Input: part model. Units: mm. Frame: model coordinates. Give positions to 0.01 mm unless a question says otherwise; leave off trailing zeros. Order: outer loops, then holes, each group sorted by start corner. A loop starts at its lowest first (then second) coordinate and runs counter-clockwise, first axis right, second up. Notation, with made-up numbers: (-8.5, 58.5) - (46.5, 58.5) arc R20 cw to (46.5, 81.5) - close; hole circle Ø9 at (8, 10). An arc over 180 degrees is marked (long way). Use a Markdown table: item, result.
from build123d import *

# Parameters (mm, degrees)
BOSS_EXTRUDE1_DEPTH      = 60
SKETCH3_W                = 20
SKETCH3_H                = 20
SKETCH3_W_2              = 18
SKETCH3_H_2              = 18
BOSS_EXTRUDE2_DEPTH      = 2000
BOSS_EXTRUDE2_DEPTH_BACK = 20
CUT_EXTRUDE1_DEPTH       = 60
SKETCH7_W                = 200
SKETCH7_H                = 200
BOSS_EXTRUDE3_DEPTH      = 4
SKETCH8_W                = 109.20231627
SKETCH8_H                = 482.966945154
CUT_EXTRUDE3_DEPTH       = 1000
CUT_EXTRUDE4_REACH       = 29
SKETCH9_R                = 3.999999996
CUT_EXTRUDE5_REACH       = 52
SKETCH10_R               = 4.000000003
CUT_EXTRUDE6_REACH       = 1055.099
SKETCH11_R               = 5
FILLET1_R                = 2
FILLET2_R                = 2


with BuildPart() as part:
    # Sketch1 → Boss-Extrude1 (new body)
    with BuildSketch(Plane(origin=(0, 0, 0), x_dir=(0, 0, -1), z_dir=(1, 0, 0))):
        Polygon((0, 0), (0, 50), (-4, 50), (-4, 4), (-27, 4), (-27, 0), align=None)
    extrude(amount=BOSS_EXTRUDE1_DEPTH)

    # Sketch3 → Boss-Extrude2 (add, two sides)
    with BuildSketch(Plane(origin=(0.734152256, 4.01424851, 2.317627458), x_dir=(0, -0.5, 0.866025404), z_dir=(-0.156434465, -0.855363194, -0.49384417))) as boss_extrude2_sk:
        with Locations((0, -29.630650218)):
            Rectangle(SKETCH3_W, SKETCH3_H)
        with Locations((0, -29.630650218)):
            Rectangle(SKETCH3_W_2, SKETCH3_H_2, mode=Mode.SUBTRACT)
    extrude(amount=BOSS_EXTRUDE2_DEPTH)
    extrude(boss_extrude2_sk.sketch, amount=-BOSS_EXTRUDE2_DEPTH_BACK)

    # Sketch5 → Cut-Extrude1 (cut)
    with BuildSketch(Plane.ZY):
        Polygon((4, 4), (4, 36.054903459), (38.781358344, 4), align=None)
    extrude(amount=-CUT_EXTRUDE1_DEPTH, mode=Mode.SUBTRACT)

    # Sketch7 → Boss-Extrude3 (add)
    with BuildSketch(Plane(origin=(-155.547262091, -982.086761679, 2e-09), x_dir=(0.987688341, -0.156434465, 0), z_dir=(0.156434465, 0.987688341, 0))):
        with Locations((5.477031178, 566.441418592)):
            Rectangle(SKETCH7_W, SKETCH7_H)
    extrude(amount=BOSS_EXTRUDE3_DEPTH)

    # Sketch8 → Cut-Extrude3 (cut)
    with BuildSketch(Plane(origin=(-155.547262091, -982.086761679, 2e-09), x_dir=(0.987688341, -0.156434465, 0), z_dir=(-0.156434465, -0.987688341, 0))):
        with Locations((4.33544583, -787.065663544)):
            Rectangle(SKETCH8_W, SKETCH8_H)
    extrude(amount=CUT_EXTRUDE3_DEPTH, mode=Mode.SUBTRACT)

    # Sketch9 → Cut-Extrude4 (cut, up to next)
    with BuildSketch(Plane(origin=(0, 0, 0), x_dir=(-1, 0, 0), z_dir=(0, 0, -1)), mode=Mode.PRIVATE) as cut_extrude4_sk1:
        with Locations((-50, 22)):
            Circle(SKETCH9_R)
    cut_extrude4_tool1 = extrude(cut_extrude4_sk1.sketch, amount=-CUT_EXTRUDE4_REACH, mode=Mode.PRIVATE) & part.part
    add(cut_extrude4_tool1.solids().sort_by_distance((50, 22, 0))[0], mode=Mode.SUBTRACT)
    # Sketch9 → Cut-Extrude4 (cut, up to next)
    with BuildSketch(Plane(origin=(0, 0, 0), x_dir=(-1, 0, 0), z_dir=(0, 0, -1)), mode=Mode.PRIVATE) as cut_extrude4_sk2:
        with Locations((-10, 22)):
            Circle(SKETCH9_R)
    cut_extrude4_tool2 = extrude(cut_extrude4_sk2.sketch, amount=-CUT_EXTRUDE4_REACH, mode=Mode.PRIVATE) & part.part
    add(cut_extrude4_tool2.solids().sort_by_distance((10, 22, 0))[0], mode=Mode.SUBTRACT)
    # Sketch9 → Cut-Extrude4 (cut, up to next)
    with BuildSketch(Plane(origin=(0, 0, 0), x_dir=(-1, 0, 0), z_dir=(0, 0, -1)), mode=Mode.PRIVATE) as cut_extrude4_sk3:
        with Locations((-10, 42)):
            Circle(SKETCH9_R)
    cut_extrude4_tool3 = extrude(cut_extrude4_sk3.sketch, amount=-CUT_EXTRUDE4_REACH, mode=Mode.PRIVATE) & part.part
    add(cut_extrude4_tool3.solids().sort_by_distance((10, 42, 0))[0], mode=Mode.SUBTRACT)
    # Sketch9 → Cut-Extrude4 (cut, up to next)
    with BuildSketch(Plane(origin=(0, 0, 0), x_dir=(-1, 0, 0), z_dir=(0, 0, -1)), mode=Mode.PRIVATE) as cut_extrude4_sk4:
        with Locations((-50, 42)):
            Circle(SKETCH9_R)
    cut_extrude4_tool4 = extrude(cut_extrude4_sk4.sketch, amount=-CUT_EXTRUDE4_REACH, mode=Mode.PRIVATE) & part.part
    add(cut_extrude4_tool4.solids().sort_by_distance((50, 42, 0))[0], mode=Mode.SUBTRACT)

    # Sketch10 → Cut-Extrude5 (cut, up to next)
    with BuildSketch(Plane.XZ, mode=Mode.PRIVATE) as cut_extrude5_sk1:
        with Locations((50, 19)):
            Circle(SKETCH10_R)
    cut_extrude5_tool1 = extrude(cut_extrude5_sk1.sketch, amount=-CUT_EXTRUDE5_REACH, mode=Mode.PRIVATE) & part.part
    add(cut_extrude5_tool1.solids().sort_by_distance((50, 0, 19))[0], mode=Mode.SUBTRACT)
    # Sketch10 → Cut-Extrude5 (cut, up to next)
    with BuildSketch(Plane.XZ, mode=Mode.PRIVATE) as cut_extrude5_sk2:
        with Locations((10, 19)):
            Circle(SKETCH10_R)
    cut_extrude5_tool2 = extrude(cut_extrude5_sk2.sketch, amount=-CUT_EXTRUDE5_REACH, mode=Mode.PRIVATE) & part.part
    add(cut_extrude5_tool2.solids().sort_by_distance((10, 0, 19))[0], mode=Mode.SUBTRACT)

    # Sketch11 → Cut-Extrude6 (cut, up to next)
    with BuildSketch(Plane(origin=(-155.547262091, -982.086761679, 2e-09), x_dir=(0.987688341, -0.156434465, 0), z_dir=(-0.156434465, -0.987688341, 0)), mode=Mode.PRIVATE) as cut_extrude6_sk1:
        with Locations((-74.522968646, -486.441418617)):
            Circle(SKETCH11_R)
    cut_extrude6_tool1 = extrude(cut_extrude6_sk1.sketch, amount=-CUT_EXTRUDE6_REACH, mode=Mode.PRIVATE) & part.part
    add(cut_extrude6_tool1.solids().sort_by_distance((-229.152729, -970.428801, -486.441419))[0], mode=Mode.SUBTRACT)
    # Sketch11 → Cut-Extrude6 (cut, up to next)
    with BuildSketch(Plane(origin=(-155.547262091, -982.086761679, 2e-09), x_dir=(0.987688341, -0.156434465, 0), z_dir=(-0.156434465, -0.987688341, 0)), mode=Mode.PRIVATE) as cut_extrude6_sk2:
        with Locations((85.477031354, -486.441418617)):
            Circle(SKETCH11_R)
    cut_extrude6_tool2 = extrude(cut_extrude6_sk2.sketch, amount=-CUT_EXTRUDE6_REACH, mode=Mode.PRIVATE) & part.part
    add(cut_extrude6_tool2.solids().sort_by_distance((-71.122595, -995.458315, -486.441419))[0], mode=Mode.SUBTRACT)
    # Sketch11 → Cut-Extrude6 (cut, up to next)
    with BuildSketch(Plane(origin=(-155.547262091, -982.086761679, 2e-09), x_dir=(0.987688341, -0.156434465, 0), z_dir=(-0.156434465, -0.987688341, 0)), mode=Mode.PRIVATE) as cut_extrude6_sk3:
        with Locations((85.477031354, -646.441418617)):
            Circle(SKETCH11_R)
    cut_extrude6_tool3 = extrude(cut_extrude6_sk3.sketch, amount=-CUT_EXTRUDE6_REACH, mode=Mode.PRIVATE) & part.part
    add(cut_extrude6_tool3.solids().sort_by_distance((-71.122595, -995.458315, -646.441419))[0], mode=Mode.SUBTRACT)
    # Sketch11 → Cut-Extrude6 (cut, up to next)
    with BuildSketch(Plane(origin=(-155.547262091, -982.086761679, 2e-09), x_dir=(0.987688341, -0.156434465, 0), z_dir=(-0.156434465, -0.987688341, 0)), mode=Mode.PRIVATE) as cut_extrude6_sk4:
        with Locations((-74.522968646, -646.441418617)):
            Circle(SKETCH11_R)
    cut_extrude6_tool4 = extrude(cut_extrude6_sk4.sketch, amount=-CUT_EXTRUDE6_REACH, mode=Mode.PRIVATE) & part.part
    add(cut_extrude6_tool4.solids().sort_by_distance((-229.152729, -970.428801, -646.441419))[0], mode=Mode.SUBTRACT)

    # Fillet1
    fillet1_edges = [part.edges().sort_by_distance(p)[0] for p in [
        (60, 50, 2),
        (60, 2, 27),
        (0, 2, 27),
        (0, 50, 2),
    ]]
    fillet(fillet1_edges, radius=FILLET1_R)

    # Fillet2
    fillet2_edges = [part.edges().sort_by_distance(p)[0] for p in [
        (-248.593627385, -965.324734939, -666.44141859),
        (-248.593627385, -965.324734938, -466.44141859),
        (-51.055959266, -996.611627945, -466.44141859),
        (-51.055959266, -996.611627945, -666.44141859),
    ]]
    fillet(fillet2_edges, radius=FILLET2_R)


solid = part.part
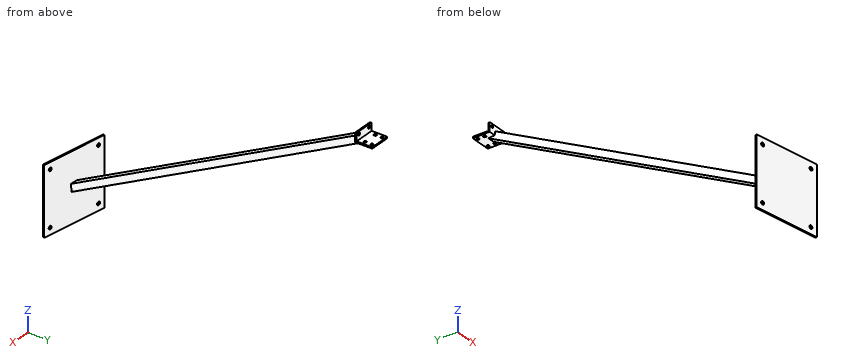
1. Section query D-D (x = -178). Return loops of the section in (y, z).
Response:
| item | result |
|---|---|
| outline | (-978.53, -666.44) - (-974.48, -666.44) - (-974.48, -466.44) - (-978.53, -466.44) - close |
2. Pin query (flat end, axial travel): pin 1 (3 mm diameter, centred on x = 32.5, z = 7.5, fed in from -Y); pin 2 (13 mm diameter, centred on x = 50, y = 42, fed in from -Z); pin 3 (5.5 mm diameter, centred on x = 27.5, y = 9.5, fed in from -Z); pin 4 (5 mm diameter, centred on x = 50, y = 22, fed in from -Z). Return the tip coordinate at first contact, or that it passes through.
Response:
| item | result |
|---|---|
| pin 1 | stops at y = -9.61 |
| pin 2 | stops at z = 0 |
| pin 3 | stops at z = -7.65 |
| pin 4 | passes through |
3. Section query B-B (z = -51). Return loops of the section in (x, y).
Response:
| item | result |
|---|---|
| outline | (0.98, -108.33) - (21.23, -108.33) - (26.71, -68.33) - (6.46, -68.33) - close; hole (2.26, -106.33) - (20.49, -106.33) - (25.43, -70.33) - (7.2, -70.33) - close |
4. Section query C-C (z = -617). Return loops of the section in (x, y), then the cut area to 3 significant figures.
Response:
| item | result |
|---|---|
| outline | (-248.91, -967.3) - (-51.37, -998.59) - (-50.74, -994.64) - (-248.28, -963.35) - close |
| area | 800 mm^2 |
5. Section query A-A (y = -321). Return loops of the section in (x, z).
Response:
| item | result |
|---|---|
| outline | (-39.75, -196.88) - (-19.5, -196.88) - (-17.67, -173.78) - (-37.92, -173.78) - close; hole (-38.64, -195.72) - (-20.42, -195.72) - (-18.77, -174.94) - (-37, -174.94) - close |
6. Material intervals for line 1 along Y through (x, z) = (50, 2.8); line 2 along Z through (x, y) = (10, 2.7); line 3 along Y through (x, z) = (-72.5, -527), sorted ascending.
Response:
| item | result |
|---|---|
| line 1 | y = 0 to 18, 26 to 38, 46 to 50 |
| line 2 | z = 0 to 15, 23 to 27 |
| line 3 | y = -995.24 to -991.19 |
